```python
from build123d import *

# Parameters (mm, degrees)
SKETCH1_R           = 36.5125
BOSS_EXTRUDE1_DEPTH = 25.4
FILLET1_R           = 12.5
SKETCH2_R           = 11
CUT_EXTRUDE1_DEPTH  = 6.5
SKETCH3_R           = 11
CUT_EXTRUDE2_DEPTH  = 6.5
SKETCH4_R           = 9
CUT_EXTRUDE3_DEPTH  = 19.9


with BuildPart() as part:
    # Sketch1 → Boss-Extrude1 (new body)
    with BuildSketch(Plane(origin=(0, 0, 0), x_dir=(1, 0, 0), z_dir=(0, 1, 0))):
        Circle(SKETCH1_R)
    extrude(amount=BOSS_EXTRUDE1_DEPTH)

    # Fillet1
    fillet1_edges = [part.edges().sort_by_distance(p)[0] for p in [
        (-36.5125, 0, 0),
        (-36.5125, 25.4, 0),
    ]]
    fillet(fillet1_edges, radius=FILLET1_R)

    # Sketch2 → Cut-Extrude1 (cut)
    with BuildSketch(Plane(origin=(0, 25.4, 0), x_dir=(1, 0, 0), z_dir=(0, 1, 0))):
        Circle(SKETCH2_R)
    extrude(amount=-CUT_EXTRUDE1_DEPTH, mode=Mode.SUBTRACT)

    # Sketch3 → Cut-Extrude2 (cut)
    with BuildSketch(Plane.XZ):
        Circle(SKETCH3_R)
    extrude(amount=-CUT_EXTRUDE2_DEPTH, mode=Mode.SUBTRACT)

    # Sketch4 → Cut-Extrude3 (cut, through all)
    with BuildSketch(Plane.XZ.offset(-6.5)):
        Circle(SKETCH4_R)
    extrude(amount=-CUT_EXTRUDE3_DEPTH, mode=Mode.SUBTRACT)


solid = part.part
```
CAD build for the part. Positions are in the model's coordinates, mm. A direction names the side the tool comes from. Round coordinates to 2 decimals unless told otherwise and drop trailing zeros. Order: outer loops, then holes, each group sorted by start corner. A loop starts at its lowest first (then second) coordinate and runs counter-clockwise, first axis right, second up. Notation, with made-up numbers: (63, 88) - (109, 88) arc R16 cw to (109, 94) - close; hole circle Ø5 at (43.5, -5). An arc over 180 degrees is marked (long way). Use CSV: the item, a comma, the result in double quotes. Start each with the question number.
1) Wall check: L1, parallel to Z at x = 0, y = 13; L2, parallel to Z at x = 0, y = 3.25; L3, parallel to X at y = 22.75, z = 0. Give the ranges that are in metal, low to high. Write a range as [from, to].
2) Two-plate mould, pull along Z, no slides. Class faces 1 (the cylindrical face through (-1.172, 12.613, 8.923)), 2 (the cylindrical face through (34.826, 12.697, -10.967)), 3 (the flat face through (10, 0, 5)): pulls with the +Z half, pulls with the -Z half, needs draft (parallel to the pull), parting line crosses it, or undercut.
3) Saw through at B-B (x = 0). List the corners of the cut face in (y, z), and give its area (3 significant figures).
4) Saw through at D-D (y = 16.75). List the corners of the cut face in (x, z).
5) Tool access for faces 4 (the flat face through (2, 6.5, -9)), 5 (the flat face through (2, 18.9, 9)), 6 (the flat face through (10, 25.4, 5)): list every direction of +Z, -Z, +X, -X, +Y, -Y with a clear straight run to the whole face (end or side of a thin tool).
6) Saw through at A-A (z = 0). List the corners of the cut face in (x, y), and give its area (3 significant figures).
7) Saw through at C-C (y = 4). List the corners of the cut face in (x, z), and give its area (3 significant figures).
8) Pin check, flat tips, straight feed: pin 1 Ø17.5 at (x, z) = (0, 0) entering from -Y; pin 2 Ø10 at (x, y) = (6, 7) entering from +Z; pin 3 Ø8 at (x, y) = (8, 2.5) entering from -Z; pin 4 Ø2 at (x, z) = (-2, 27.5) entering from -Y (3 decimals). Stop position of each tip, or through.
Values follow:
1,L1,"z = [-36.51, -9], [9, 36.51]"
1,L2,"z = [-32.42, -11], [11, 32.42]"
1,L3,"x = [-31.71, -11], [11, 31.71]"
2,face 1,"undercut"
2,face 2,"parting line crosses it"
2,face 3,"needs draft"
3,outline,"(0, -24.01) arc R12.5 ccw to (12.5, -36.51) - (12.9, -36.51) arc R12.5 ccw to (25.4, -24.01) - (25.4, -11) - (18.9, -11) - (18.9, -9) - (6.5, -9) - (6.5, -11) - (0, -11) - close; (0, 11) - (6.5, 11) - (6.5, 9) - (18.9, 9) - (18.9, 11) - (25.4, 11) - (25.4, 24.01) arc R12.5 ccw to (12.9, 36.51) - (12.5, 36.51) arc R12.5 ccw to (0, 24.01) - close"
3,area,"1,210 mm2"
4,outline,"circle Ø71.81 at (0, 0); hole circle Ø18 at (0, 0)"
5,face 4,"-Y"
5,face 5,"+Y"
5,face 6,"+Z, -Z, +X, -X, +Y"
6,outline,"(-36.51, 12.5) arc R12.5 ccw to (-24.01, 0) - (-11, 0) - (-11, 6.5) - (-9, 6.5) - (-9, 18.9) - (-11, 18.9) - (-11, 25.4) - (-24.01, 25.4) arc R12.5 ccw to (-36.51, 12.9) - close; (9, 6.5) - (11, 6.5) - (11, 0) - (24.01, 0) arc R12.5 ccw to (36.51, 12.5) - (36.51, 12.9) arc R12.5 ccw to (24.01, 25.4) - (11, 25.4) - (11, 18.9) - (9, 18.9) - close"
6,area,"1,210 mm2"
7,outline,"circle Ø66.36 at (0, 0); hole circle Ø22 at (0, 0)"
7,area,"3,080 mm2"
8,pin 1,"passes through"
8,pin 2,"stops at z = 36.3"
8,pin 3,"stops at z = -34.21"
8,pin 4,"stops at y = 0.265"
